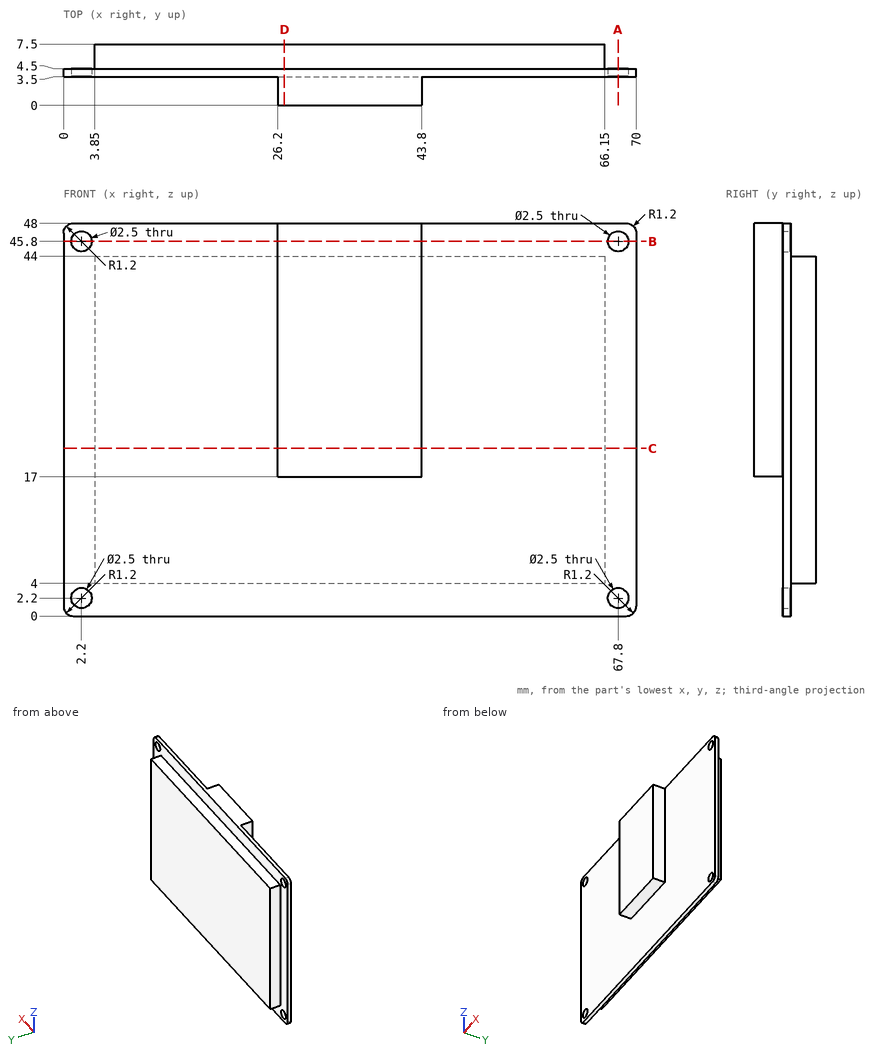
For this review, use the dimensioned drawing (mm, ordinates from the lowest corner) and the shaded views. Round coordinates to 2 decimals unless told otherwise and drop trailing zeros. Order: outer loops, then holes, each group sorted by start corner. A loop starts at its lowest first (then second) coordinate and runs counter-clockwise, first axis right, second up.
1) Consider section C-C (z = 20.5). State the section outline as (x, y) points.
The answers:
outline: (0, 3.5) - (26.2, 3.5) - (26.2, 0) - (43.8, 0) - (43.8, 3.5) - (70, 3.5) - (70, 4.5) - (66.15, 4.5) - (66.15, 7.5) - (3.85, 7.5) - (3.85, 4.5) - (0, 4.5) - close
2) Consider section A-A (x = 67.8). State the section outline as (y, z) points.
The answers:
outline: (3.5, 0) - (4.5, 0) - (4.5, 0.95) - (3.5, 0.95) - close; (3.5, 3.45) - (4.5, 3.45) - (4.5, 44.55) - (3.5, 44.55) - close; (3.5, 47.05) - (4.5, 47.05) - (4.5, 48) - (3.5, 48) - close
3) For L1, parallel to X at y = 4.2, z = 45.8; L2, parallel to Y at x = 47, z = 39; L3, parallel to X at y = 7.25, z = 29.5, list the stretches that pass through material, from the lowest coordinate up.
The answers:
L1: x = 0 to 0.95, 3.45 to 66.55, 69.05 to 70
L2: y = 3.5 to 7.5
L3: x = 3.85 to 66.15
4) Consider section B-B (z = 45.8). State the section outline as (x, y) points.
The answers:
outline: (0, 3.5) - (0.95, 3.5) - (0.95, 4.5) - (0, 4.5) - close; (3.45, 3.5) - (26.2, 3.5) - (26.2, 0) - (43.8, 0) - (43.8, 3.5) - (66.55, 3.5) - (66.55, 4.5) - (3.45, 4.5) - close; (69.05, 3.5) - (70, 3.5) - (70, 4.5) - (69.05, 4.5) - close
5) Clearance check with flat-ended pins moving along their axes: pin 1 Ø3.5 at (x, y) = (45.5, 6.5) entering from -Z; pin 2 Ø1 at (x, z) = (24.5, 18.5) entering from -Y; pin 3 Ø3 at (x, z) = (2.2, 45.8) entering from +Y. State where each tip first meets the part, or that it passes through.
The answers:
pin 1: stops at z = 4
pin 2: stops at y = 3.5
pin 3: stops at y = 4.5
6) Consider section D-D (x = 27). State the section outline as (y, z) points.
The answers:
outline: (0, 17) - (3.5, 17) - (3.5, 0) - (4.5, 0) - (4.5, 4) - (7.5, 4) - (7.5, 44) - (4.5, 44) - (4.5, 48) - (0, 48) - close
